Check sheet for the modelled part. Datum: model origin and axes. Units: mm. A direction names the side the tool comes from. Coordinates: 2 decimals unless noted, no trailing zeros. Order: outer loops, then holes, each group sorted by start corner. A loop starts at its lowest first (then second) coordinate and runs counter-clockwise, first axis right, second up. Notation, with made-up numbers: M 0,63.25 L 55,63.25 A15 cw 55,73.25 Z; hole C 83.5,32 d2. An arc over 180 degrees is marked long. Answer in a Markdown table with one row per item. Add a question column.
from build123d import *

# Parameters (mm, degrees)
SKETCH_1_W          = 13
SKETCH_1_H          = 22
SKETCH_1_R          = 2.2
SKETCH_1_H_2        = 19
SKETCH_1_H_3        = 15
SKETCH_1_W_2        = 104
EXTRUDE_3_DEPTH     = 2
SKETCH_2_R          = 2.25
CUT_EXTRUDE_1_DEPTH = 10
CUT_EXTRUDE_2_DEPTH = 10
SKETCH_4_W          = 104
SKETCH_4_H          = 4
CUT_EXTRUDE_3_DEPTH = 10
FILLET_1_R          = 2
FILLET_2_R          = 3


with BuildPart() as part:
    # 草图1 → 凸台-拉伸3 (new body)
    # profile 1 of 8: a face of its own
    with BuildSketch(Plane(origin=(0, 0, 0), x_dir=(1, 0, 0), z_dir=(0, 1, 0))):
        with Locations((6.5, -45)):
            Rectangle(SKETCH_1_W, SKETCH_1_H)
        with Locations(Location((7.5, -37.5, 0), (0, 0, 270))):
            Circle(SKETCH_1_R, mode=Mode.SUBTRACT)
    # profile 2 of 8: a face of its own
    with BuildSketch(Plane(origin=(0, 0, 0), x_dir=(1, 0, 0), z_dir=(0, 1, 0))):
        with Locations((6.5, -24.5)):
            Rectangle(SKETCH_1_W, SKETCH_1_H_2)
    # profile 3 of 8: a face of its own
    with BuildSketch(Plane(origin=(0, 0, 0), x_dir=(1, 0, 0), z_dir=(0, 1, 0))):
        with Locations((6.5, -7.5)):
            Rectangle(SKETCH_1_W, SKETCH_1_H_3)
        with Locations(Location((7.5, -7.5, 0), (0, 0, 270))):
            Circle(SKETCH_1_R, mode=Mode.SUBTRACT)
    # profile 4 of 8: a face of its own
    with BuildSketch(Plane(origin=(0, 0, 0), x_dir=(1, 0, 0), z_dir=(0, 1, 0))):
        with Locations((65, -7.5)):
            Rectangle(SKETCH_1_W_2, SKETCH_1_H_3)
        with Locations(Location((45.75, -7.5, 0), (0, 0, 270))):
            Circle(SKETCH_1_R, mode=Mode.SUBTRACT)
        with Locations(Location((84.25, -7.5, 0), (0, 0, 270))):
            Circle(SKETCH_1_R, mode=Mode.SUBTRACT)
    # profile 5 of 8: a face of its own
    with BuildSketch(Plane(origin=(0, 0, 0), x_dir=(1, 0, 0), z_dir=(0, 1, 0))):
        with Locations((123.5, -7.5)):
            Rectangle(SKETCH_1_W, SKETCH_1_H_3)
        with Locations(Location((122.5, -7.5, 0), (0, 0, 270))):
            Circle(SKETCH_1_R, mode=Mode.SUBTRACT)
    # profile 6 of 8: a face of its own
    with BuildSketch(Plane(origin=(0, 0, 0), x_dir=(1, 0, 0), z_dir=(0, 1, 0))):
        with Locations((123.5, -24.5)):
            Rectangle(SKETCH_1_W, SKETCH_1_H_2)
    # profile 7 of 8: a face of its own
    with BuildSketch(Plane(origin=(0, 0, 0), x_dir=(1, 0, 0), z_dir=(0, 1, 0))):
        with Locations((123.5, -45)):
            Rectangle(SKETCH_1_W, SKETCH_1_H)
        with Locations(Location((122.5, -37.5, 0), (0, 0, 270))):
            Circle(SKETCH_1_R, mode=Mode.SUBTRACT)
    # profile 8 of 8: a face of its own
    with BuildSketch(Plane(origin=(0, 0, 0), x_dir=(1, 0, 0), z_dir=(0, 1, 0))):
        with Locations((65, -24.5)):
            Rectangle(SKETCH_1_W_2, SKETCH_1_H_2)
    extrude(amount=EXTRUDE_3_DEPTH)

    # 草图2 → 切除-拉伸1 (cut)
    with BuildSketch(Plane(origin=(0, 2, 0), x_dir=(1, 0, 0), z_dir=(0, 1, 0))):
        with Locations(Location((38, -20, 0), (0, 0, 270))):
            Circle(SKETCH_2_R)
        with Locations(Location((92, -20, 0), (0, 0, 270))):
            Circle(SKETCH_2_R)
    extrude(amount=-CUT_EXTRUDE_1_DEPTH, mode=Mode.SUBTRACT)

    # 草图3 → 切除-拉伸2 (cut)
    with BuildSketch(Plane(origin=(0, 2, 0), x_dir=(1, 0, 0), z_dir=(0, 1, 0))):
        with BuildLine():
            ThreePointArc((38.443762995, -4), (40.191298213, -5.02731266), (40.143568379, -7.053879338))
            Line((40.143568379, -7.053879338), (28.817131634, -25.3223257))
            ThreePointArc((28.817131634, -25.3223257), (27.096125533, -26.268333991), (25.39556113, -25.286053787))
            Line((25.39556113, -25.286053787), (14.598439949, -7.017607424))
            ThreePointArc((14.598439949, -7.017607424), (14.583078872, -5.00884281), (16.320205069, -4))
            Line((16.320205069, -4), (38.443762995, -4))
        make_face()
        with BuildLine():
            Line((3.788738097, -15.906719656), (3.788738097, -25))
            ThreePointArc((3.788738097, -25), (4.374524535, -26.414213562), (5.788738097, -27))
            Line((5.788738097, -27), (15.89527198, -27))
            ThreePointArc((15.89527198, -27), (18.500961276, -25.486735785), (18.477919661, -22.473588863))
            Line((18.477919661, -22.473588863), (13.093150898, -13.362701095))
            ThreePointArc((13.093150898, -13.362701095), (7.470038739, -11.083750445), (3.788738097, -15.906719656))
        make_face()
        with BuildLine():
            Line((65, -27), (65, -6))
            Line((65, -6), (54.809846331, -6))
            ThreePointArc((54.809846331, -6), (53.873365064, -6.23279802), (53.154894782, -6.876997163))
            Line((53.154894782, -6.876997163), (41.619180496, -23.876997163))
            ThreePointArc((41.619180496, -23.876997163), (41.506930066, -25.936481267), (43.274132045, -27))
            Line((43.274132045, -27), (65, -27))
        make_face()
        with BuildLine():
            Line((75.190153669, -6), (65, -6))
            Line((65, -6), (65, -27))
            Line((65, -27), (86.725867955, -27))
            ThreePointArc((86.725867955, -27), (88.493069934, -25.936481267), (88.380819504, -23.876997163))
            Line((88.380819504, -23.876997163), (76.845105218, -6.876997163))
            ThreePointArc((76.845105218, -6.876997163), (76.126634936, -6.23279802), (75.190153669, -6))
        make_face()
        with BuildLine():
            Line((89.856431621, -7.053879338), (101.182868366, -25.3223257))
            ThreePointArc((101.182868366, -25.3223257), (102.903874467, -26.268333991), (104.60443887, -25.286053787))
            Line((104.60443887, -25.286053787), (115.401560051, -7.017607424))
            ThreePointArc((115.401560051, -7.017607424), (115.416921128, -5.00884281), (113.679794931, -4))
            Line((113.679794931, -4), (91.556237005, -4))
            ThreePointArc((91.556237005, -4), (89.808701787, -5.02731266), (89.856431621, -7.053879338))
        make_face()
        with BuildLine():
            ThreePointArc((126.211261903, -25), (125.625475465, -26.414213562), (124.211261903, -27))
            Line((124.211261903, -27), (114.10472802, -27))
            ThreePointArc((114.10472802, -27), (111.499038724, -25.486735785), (111.522080339, -22.473588863))
            Line((111.522080339, -22.473588863), (116.906849102, -13.362701095))
            ThreePointArc((116.906849102, -13.362701095), (122.529961261, -11.083750445), (126.211261903, -15.906719656))
            Line((126.211261903, -15.906719656), (126.211261903, -25))
        make_face()
    extrude(amount=-CUT_EXTRUDE_2_DEPTH, mode=Mode.SUBTRACT)

    # 草图4 → 切除-拉伸3 (cut)
    with BuildSketch(Plane(origin=(0, 2, 0), x_dir=(1, 0, 0), z_dir=(0, 1, 0))):
        with Locations((65, -32)):
            Rectangle(SKETCH_4_W, SKETCH_4_H)
    extrude(amount=-CUT_EXTRUDE_3_DEPTH, mode=Mode.SUBTRACT)

    # 圆角1
    fillet_1_edges = [part.edges().sort_by_distance(p)[0] for p in [
        (13, 1, 30),
        (117, 1, 30),
    ]]
    fillet(fillet_1_edges, radius=FILLET_1_R)

    # 圆角2
    fillet_2_edges = [part.edges().sort_by_distance(p)[0] for p in [
        (130, 1, 56),
        (117, 1, 56),
        (13, 1, 56),
        (0, 1, 56),
        (0, 1, 0),
        (130, 1, 0),
    ]]
    fillet(fillet_2_edges, radius=FILLET_2_R)


solid = part.part
1. Set-up check for faces 4 (the flat face through (47.468, 1.014, 15.258)), 5 (the cylindrical face through (117.86, 1.01, 55.1)), 6 (the cylindrical face through (0.9, 1.01, 55.14)): record each of +Z, -Z, +X, -X, +Y, -Y from which the full face is reachable in a straight line by a thin tool's end or side.
2. Go/stop test with flat-tipped pins: pin 1 Ø3.5 at (x, z) = (122.5, 7.5) entering from +Y; pin 2 Ø0.6 at (x, y) = (107, 1) entering from +Z. Record where each tip stops, or that it passes through.
3. Section check A-A on z = 42.5. Enter the section's corners in (x, y), then the cut area to 3 significant figures.
4. Section check C-C on x = 45.75. Enter the section's corners in (y, z).
5. Scan lines: line 1 (X direction, y = 0.3, z = 50); line 2 (Z direction, x = 86, y = 0.5); line 3 (Z direction, x = 68.5, y = 0.4). Record each from-to range of solid material in increasing order.
6. Release check for a two-part mould opening along Z. For faces 1 (the flat face through (64, 2, 28)), 2 (the cylindrical face through (129.14, 1.01, 55.1)), 3 (the flat face through (15.82, 1.01, 17.98)) record: released by +Z, released by -Z, zero draft, split by the parting line, or undercut.
7. Section check B-B on x = 72. Enter the section's corners in (y, z).
8. Section check D-D on z = 20. State how many separate pieces and enclosed holes the cut face has, then the cut area to 3 significant figures.
Result sheet:
| question | item | result |
|---|---|---|
| 1 | face 4 | +Y, -Y |
| 1 | face 5 | +Z, +Y, -Y |
| 1 | face 6 | +Z, -X, +Y, -Y |
| 2 | pin 1 | through |
| 2 | pin 2 | z = 30 |
| 3 | outline | M 0,0 L 13,0 L 13,2 L 0,2 Z; M 117,0 L 130,0 L 130,2 L 117,2 Z |
| 3 | area | 52.0 mm^2 |
| 4 | outline | M 0,0 L 2,0 L 2,5.3 L 0,5.3 Z; M 0,9.7 L 2,9.7 L 2,17.79 L 0,17.79 Z; M 0,27 L 2,27 L 2,30 L 0,30 Z |
| 5 | line 1 | 0 to 13, 117 to 130 |
| 5 | line 2 | 0 to 6.17, 8.83 to 20.37, 27 to 30 |
| 5 | line 3 | 0 to 6, 27 to 30 |
| 6 | face 1 | zero draft |
| 6 | face 2 | released by +Z |
| 6 | face 3 | undercut |
| 7 | outline | M 0,0 L 2,0 L 2,6 L 0,6 Z; M 0,27 L 2,27 L 2,30 L 0,30 Z |
| 8 | separate pieces | 8 |
| 8 | enclosed holes | 0 |
| 8 | area | 66.7 mm^2 |
